The listing builds one solid part. Answer for the finished solid, in the listing's coordinates (mm). Face numbers are marked on the shaded views. A direction names the side the tool comes from. Round coordinates to 2 decimals unless told otherwise and drop trailing zeros. Write each loop counter-clockwise with the first axis right and the second up, starting at its lowest first coordinate (ties: lowest second). Pieces come first, ordered by that corner, then holes. Notation, with made-up numbers: (-30.75, 77.25) - (-17.75, 77.25) arc R25 ccw to (-17.75, 94.25) - close; hole circle Ø6 at (58, -17). An arc over 180 degrees is marked (long way). Answer in a Markdown table with one row per item.
from build123d import *

# Parameters (mm, degrees)
SKIZZE1_R                        = 18
AUFSATZ_LINEAR_AUSTRAGEN1_DEPTH  = 10
SKIZZE2_OUTSIDE_W                = 48.376
SKIZZE2_OUTSIDE_H                = 48.376
SKIZZE2_OUTSIDE_W_2              = 36
SKIZZE2_OUTSIDE_H_2              = 27.5
SCHNITT_LINEAR_AUSTRAGEN1_DEPTH  = 10
SCHNITT_LINEAR_AUSTRAGEN2_DEPTH  = 10
SKIZZE4_R                        = 3
SCHNITT_LINEAR_AUSTRAGEN3_DEPTH  = 22.5
M3_GEWINDEBOHRUNG1_D             = 2.5
F_3_5_3_5_DURCHMESSER_BOHRUNG1_D = 3.5
SKIZZE9_R                        = 0.75
SCHNITT_LINEAR_AUSTRAGEN4_DEPTH  = 10
VERRUNDUNG1_R                    = 0.6


with BuildPart() as part:
    # Skizze1 → Aufsatz-Linear austragen1 (new body)
    with BuildSketch(Plane(origin=(0, 0, 0), x_dir=(1, 0, 0), z_dir=(0, 1, 0))):
        with Locations(Location((0, 0, 0), (0, 0, 270))):
            Circle(SKIZZE1_R)
    extrude(amount=AUFSATZ_LINEAR_AUSTRAGEN1_DEPTH)

    # Skizze2 outside → Schnitt-Linear austragen1 (cut)
    with BuildSketch(Plane(origin=(0, 10, 0), x_dir=(1, 0, 0), z_dir=(0, 1, 0))):
        Rectangle(SKIZZE2_OUTSIDE_W, SKIZZE2_OUTSIDE_H)
        Rectangle(SKIZZE2_OUTSIDE_W_2, SKIZZE2_OUTSIDE_H_2, mode=Mode.SUBTRACT)
    extrude(amount=-SCHNITT_LINEAR_AUSTRAGEN1_DEPTH, mode=Mode.SUBTRACT)

    # Skizze3 → Schnitt-Linear austragen2 (cut)
    with BuildSketch(Plane(origin=(0, 10, 0), x_dir=(1, 0, 0), z_dir=(0, 1, 0))):
        Polygon((2.886751346, 5), (-2.886751346, 5), (-5.773502692, 0), (-2.886751346, -5), (2.886751346, -5), (5.773502692, 0), align=None)
    extrude(amount=-SCHNITT_LINEAR_AUSTRAGEN2_DEPTH, mode=Mode.SUBTRACT)

    # Skizze4 → Schnitt-Linear austragen3 (cut, symmetric)
    with BuildSketch(Plane(origin=(0, 0, 0), x_dir=(0, 0, -1), z_dir=(1, 0, 0))):
        with Locations((0, 10)):
            Circle(SKIZZE4_R)
    extrude(amount=SCHNITT_LINEAR_AUSTRAGEN3_DEPTH, both=True, mode=Mode.SUBTRACT)

    # M3 Gewindebohrung1 (through all)
    with Locations(Plane(origin=(0, 10, 0), x_dir=(1, 0, 0), z_dir=(0, 1, 0))):
        with Locations((0, 10.9), (0, -10.9)):
            Hole(M3_GEWINDEBOHRUNG1_D / 2)

    # Ø3.5 (3.5) Durchmesser Bohrung1 (through all)
    with Locations(Plane(origin=(0, 10, 0), x_dir=(1, 0, 0), z_dir=(0, 1, 0))):
        with Locations((-10.9, 10.9), (10.9, 10.9), (10.9, -10.9), (-10.9, -10.9)):
            Hole(F_3_5_3_5_DURCHMESSER_BOHRUNG1_D / 2)

    # Skizze9 → Schnitt-Linear austragen4 (cut)
    with BuildSketch(Plane(origin=(0, 10, 0), x_dir=(1, 0, 0), z_dir=(0, 1, 0))):
        with Locations((-2.886751346, 5)):
            Circle(SKIZZE9_R)
        with Locations((2.886751346, 5)):
            Circle(SKIZZE9_R)
        with Locations((5.773502692, 0)):
            Circle(SKIZZE9_R)
        with Locations((2.886751346, -5)):
            Circle(SKIZZE9_R)
        with Locations((-2.886751346, -5)):
            Circle(SKIZZE9_R)
        with Locations((-5.773502692, 0)):
            Circle(SKIZZE9_R)
    extrude(amount=-SCHNITT_LINEAR_AUSTRAGEN4_DEPTH, mode=Mode.SUBTRACT)

    # Verrundung1
    # the kernel refuses this fillet: 0.6 mm, written as the material it takes off along each edge
    with BuildSketch(Plane(origin=(5.398502692, -1.148346656, -0.649519053), x_dir=(-0.4999999999999986, 0, -0.8660254037844394), z_dir=(0, 1, 0))) as verrundung1_piece_1:
        with BuildLine():
            CenterArc((0.459338662, -0.6), VERRUNDUNG1_R, 90, 63.612200039)
            ThreePointArc((-0.078145188, -0.333333333), (-0.019797593, -0.171185412), (0, 0))
            Line((0, 0), (0.459338662, 0))
        make_face()
    extrude(amount=9.367849683, mode=Mode.SUBTRACT)
    with BuildSketch(Plane(origin=(5.398502692, -1.148346656, 0.649519053), x_dir=(0.9572887202141677, 0, 0.2891337167310671), z_dir=(0, 1, 0))) as verrundung1_piece_2:
        with BuildLine():
            CenterArc((0.479319154, -0.584161925), VERRUNDUNG1_R, 103.193899981, 63.612200039)
            Line((-0.104842771, -0.447213595), (0, 0))
            ThreePointArc((0, 0), (0.171185412, -0.019797593), (0.342370824, 0))
        make_face()
    extrude(amount=9.367849683, mode=Mode.SUBTRACT)
    with BuildSketch(Plane(origin=(3.261751346, -1.148346656, 4.350480947), x_dir=(0.5000000000000002, 0, -0.8660254037844385), z_dir=(0, 1, 0)), Plane(origin=(-3.261751346, -1.148346656, -4.350480947), x_dir=(-0.5000000000000006, 0, 0.8660254037844383), z_dir=(0, 1, 0)), Plane(origin=(2.136751346, -1.148346656, -5), x_dir=(-1, 0, 0), z_dir=(0, 1, 0))) as verrundung1_piece_3:
        with BuildLine():
            CenterArc((0.459338662, -0.6), VERRUNDUNG1_R, 90, 63.612200039)
            ThreePointArc((-0.078145188, -0.333333333), (-0.019797593, -0.171185412), (0, 0))
            Line((0, 0), (0.459338662, 0))
        make_face()
    extrude(amount=12.296693311, mode=Mode.SUBTRACT)
    with BuildSketch(Plane(origin=(2.136751346, -1.148346656, 5), x_dir=(0.22824721632736691, 0, 0.9736032088272965), z_dir=(0, 1, 0)), Plane(origin=(-3.261751346, -1.148346656, 4.350480947), x_dir=(-0.7290415038868022, 0, 0.684469492096229), z_dir=(0, 1, 0)), Plane(origin=(3.261751346, -1.148346656, -4.350480947), x_dir=(0.7290415038868017, 0, -0.6844694920962296), z_dir=(0, 1, 0))) as verrundung1_piece_4:
        with BuildLine():
            CenterArc((0.479319154, -0.584161925), VERRUNDUNG1_R, 103.193899981, 63.612200039)
            Line((-0.104842771, -0.447213595), (0, 0))
            ThreePointArc((0, 0), (0.171185412, -0.019797593), (0.342370824, 0))
        make_face()
    extrude(amount=12.296693311, mode=Mode.SUBTRACT)
    with BuildSketch(Plane(origin=(-2.136751346, 11.148346656, 5), x_dir=(1, 0, 0), z_dir=(0, -1, 0))) as verrundung1_piece_5:
        with BuildLine():
            CenterArc((0.459338662, 0.6), VERRUNDUNG1_R, 206.387799961, 63.612200039)
            ThreePointArc((-0.078145188, 0.333333333), (-0.019797593, 0.171185412), (0, 0))
            Line((0, 0), (0.459338662, 0))
        make_face()
    extrude(amount=12.296693311, mode=Mode.SUBTRACT)
    with BuildSketch(Plane(origin=(-5.398502692, -1.148346656, 0.649519053), x_dir=(-0.9572887202141677, 0, 0.2891337167310672), z_dir=(0, 1, 0))) as verrundung1_piece_6:
        with BuildLine():
            CenterArc((0.479319154, 0.584161925), VERRUNDUNG1_R, 193.193899981, 63.612200039)
            Line((-0.104842771, 0.447213595), (0, 0))
            ThreePointArc((0, 0), (0.171185412, 0.019797593), (0.342370824, 0))
        make_face()
    extrude(amount=9.367849683, mode=Mode.SUBTRACT)
    with BuildSketch(Plane(origin=(-5.398502692, -1.148346656, -0.649519053), x_dir=(0.5000000000000002, 0, -0.8660254037844385), z_dir=(0, 1, 0))) as verrundung1_piece_7:
        with BuildLine():
            CenterArc((0.459338662, 0.6), VERRUNDUNG1_R, 206.387799961, 63.612200039)
            ThreePointArc((-0.078145188, 0.333333333), (-0.019797593, 0.171185412), (0, 0))
            Line((0, 0), (0.459338662, 0))
        make_face()
    extrude(amount=9.367849683, mode=Mode.SUBTRACT)
    with BuildSketch(Plane(origin=(-2.136751346, 11.148346656, -5), x_dir=(-0.22824721632736567, 0, -0.9736032088272967), z_dir=(0, -1, 0))) as verrundung1_piece_8:
        with BuildLine():
            CenterArc((0.479319154, 0.584161925), VERRUNDUNG1_R, 193.193899981, 63.612200039)
            Line((-0.104842771, 0.447213595), (0, 0))
            ThreePointArc((0, 0), (0.171185412, 0.019797593), (0.342370824, 0))
        make_face()
    extrude(amount=12.296693311, mode=Mode.SUBTRACT)


solid = part.part
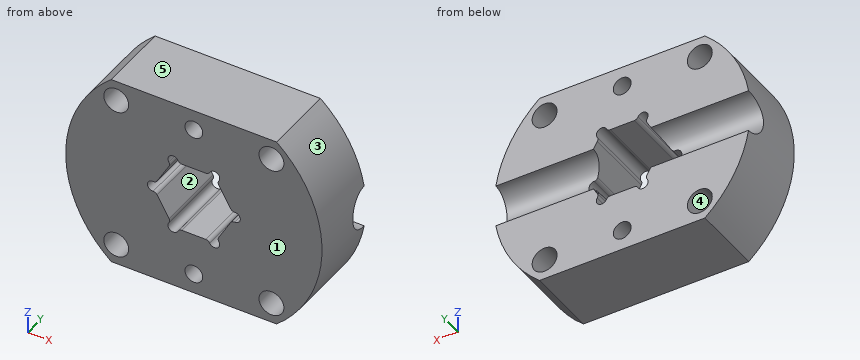
(1) Find the intervals of material crossed by line 1 (Z direction, x = -10.9, y = 4); line 2 (Z direction, x = 0, y = 7.5); line 3 (Z direction, x = -10.9, y = 8.25), in increasing order.
Checked values:
| item | result |
|---|---|
| line 1 | z = -13.75 to -12.65, -9.15 to 9.15, 12.65 to 13.75 |
| line 2 | z = -13.75 to -12.15, -9.65 to -5, 5 to 9.65, 12.15 to 13.75 |
| line 3 | z = -13.75 to -12.65, -9.15 to -2.44, 2.44 to 9.15, 12.65 to 13.75 |
(2) Flat-ended cylindrical pins translate along their axes: pin 1 (1.5 mm diameter, centred on y = 1, z = -3.5, fed in from -X); pin 2 (6 mm diameter, centred on y = 2.5, z = -4.5, fed in from +X). Find the tip coordinate at first contact, or state that the pin passes through.
Checked values:
| item | result |
|---|---|
| pin 1 | stops at x = -17.79 |
| pin 2 | stops at x = 17.94 |
(3) Section B-B (z = 0) is taken. Give the vertices of the cut face in (x, y).
Checked values:
| item | result |
|---|---|
| outline | (-18, 0) - (-6.52, 0) - (-6.52, 7) - (-18, 7) - close; (6.52, 0) - (18, 0) - (18, 7) - (6.52, 7) - close |
(4) For the marked faces 1 and 2, determine the directions among +Z, -Z, +X, -X, +Y, -Y from which every point of the face is accessible in a straight line to the end or side of a thin tool.
Checked values:
| item | result |
|---|---|
| face 1 | +Z, -Z, +X, -X, -Y |
| face 2 | +Y, -Y |
(5) Section C-C (y = 8) is taken. State how many separate pieces and enclosed holes the cut face has, and give its area (3 significant figures).
Checked values:
| item | result |
|---|---|
| separate pieces | 2 |
| enclosed holes | 6 |
| area | 628 mm2 |
(6) Section D-D (x = 0) is taken. Give the vertices of the cut face in (y, z).
Checked values:
| item | result |
|---|---|
| outline | (0, -13.75) - (10, -13.75) - (10, -12.15) - (0, -12.15) - close; (0, -9.65) - (10, -9.65) - (10, -5) - (0, -5) - close; (0, 5) - (10, 5) - (10, 9.65) - (0, 9.65) - close; (0, 12.15) - (10, 12.15) - (10, 13.75) - (0, 13.75) - close |
(7) Section A-A (x = 10.9) is taken. Give the vertices of the cut face in (y, z), and give its area (3 significant figures).
Checked values:
| item | result |
|---|---|
| outline | (0, -13.75) - (10, -13.75) - (10, -12.65) - (0, -12.65) - close; (0, -9.15) - (10, -9.15) - (10, -3) arc R3 cw to (10, 3) - (10, 9.15) - (0, 9.15) - close; (0, 12.65) - (10, 12.65) - (10, 13.75) - (0, 13.75) - close |
| area | 191 mm2 |
(8) For a pull along Z with two mould halves and no side action, classify the marked faces 3, 4 and 5 as pulls with the +Z half, pulls with the -Z half, needs draft (parallel to the pull), parting line crosses it, or undercut.
Checked values:
| item | result |
|---|---|
| face 3 | parting line crosses it |
| face 4 | undercut |
| face 5 | pulls with the +Z half |
